Read the model definition and answer for the solid it produces. Units are mm, in the model's axes. A direction names the side the tool comes from. Round coordinates to 2 decimals unless told otherwise and drop trailing zeros. Write each loop counter-clockwise with the first axis right and the second up, starting at its lowest first coordinate (ties: lowest second). Pieces come first, ordered by that corner, then holes. Notation, with made-up numbers: (79.25, 60) -> (85.25, 60) arc R20 cw to (85.25, 65) -> close; hole circle Ø4 at (49.25, -21). An arc over 180 degrees is marked (long way). Return JSON: item names as keys, results as strings.
from build123d import *

# Parameters (mm, degrees)
F1_DEPTH = 12
F2_R     = 2.75
F3_DEPTH = 12.001


with BuildPart() as f1:
    # F0 (on Top) → F1 (new body)
    with BuildSketch(Plane.XY):
        Polygon((0, 12), (0, 0), (0, -30), (12, -30), (12, 0), (58, 0), (58, 70), (46, 70), (46, 12), align=None)
    extrude(amount=F1_DEPTH)

    # F2 (on face) → F3 (cut, through all)
    with BuildSketch(Plane.YZ.offset(12)):
        with Locations((-24, 6)):
            Circle(F2_R)
        with Locations((-8, 6)):
            Circle(F2_R)
    extrude(amount=-F3_DEPTH, mode=Mode.SUBTRACT)


solid = f1.part
Item 1: Flat-ended cylindrical pins translate along their axes: pin 1 (3.5 mm diameter, centred on x = 24.5, z = 3.5, fed in from -Y); pin 2 (6 mm diameter, centred on y = -13, z = 5.5, fed in from +X); pin 3 (1 mm diameter, centred on x = 12.5, z = 8, fed in from +Y). Find the tip coordinate at first contact, or state that the pin passes through.
Worked answers:
{"pin 1": "stops at y = 0", "pin 2": "stops at x = 12", "pin 3": "stops at y = 12"}
Item 2: For a pull along Z with two mould halves and no side action, classify faces 4 (the flat face through (0, -9, 3)), 5 (the cylindrical face through (6.084, -26.747, 6.121)), 6 (the flat face through (33, 9, 12)), 7 (the flat face through (33, 9, 0)) as released by +Z, released by -Z, zero draft, split by the parting line, or undercut.
Worked answers:
{"face 4": "zero draft", "face 5": "undercut", "face 6": "released by +Z", "face 7": "released by -Z"}
Item 3: Section C-C (x = 5.5) is taken. Give the vertices of the cut face in (y, z), then the cut area to 3 significant figures.
Worked answers:
{"outline": "(-30, 0) -> (12, 0) -> (12, 12) -> (-30, 12) -> close; hole circle Ø5.5 at (-24, 6); hole circle Ø5.5 at (-8, 6)", "area": "456 mm2"}
Item 4: Section D-D (z = 1.75) is taken. Give the vertices of the cut face in (x, y).
Worked answers:
{"outline": "(0, -30) -> (12, -30) -> (12, 0) -> (58, 0) -> (58, 70) -> (46, 70) -> (46, 12) -> (0, 12) -> close"}
Item 5: Section A-A (y = -8) is taken. Give the vertices of the cut face in (x, z).
Worked answers:
{"outline": "(0, 0) -> (12, 0) -> (12, 3.25) -> (0, 3.25) -> close; (0, 8.75) -> (12, 8.75) -> (12, 12) -> (0, 12) -> close"}
Item 6: Section B-B (z = 6) is taken. Give the vertices of the cut face in (x, y).
Worked answers:
{"outline": "(0, -30) -> (12, -30) -> (12, -26.75) -> (0, -26.75) -> close; (0, -21.25) -> (12, -21.25) -> (12, -10.75) -> (0, -10.75) -> close; (0, -5.25) -> (12, -5.25) -> (12, 0) -> (58, 0) -> (58, 70) -> (46, 70) -> (46, 12) -> (0, 12) -> close"}
Item 7: Straight lines are drawn through the part: L1, parallel to Z at x = 8, y = -24; L2, parallel to X at y = 66, z = 4.75; L3, parallel to Y at x = 22.5, z = 5.5. For each, find the intervals that lie inside material, in ascending order. Write a range as [from, to].
Worked answers:
{"L1": "z = [0, 3.25], [8.75, 12]", "L2": "x = [46, 58]", "L3": "y = [0, 12]"}
Item 8: A tool of negligible diameter and unlimited length cuts with its end or side. For faces 1 (the flat face through (12, -15, 6)), 2 (the flat face through (46, 41, 6)), 3 (the cylindrical face through (6.08, -6.73, 3.56)), from which of +Z, -Z, +X, -X, +Y, -Y can it reach the whole face along a straight path? Write none if from no direction.
Worked answers:
{"face 1": "+Z, -Z, +X, -Y", "face 2": "+Z, -Z, -X, +Y", "face 3": "+X, -X"}
